from build123d import *

# Parameters (mm, degrees)
SKETCH1_R           = 200
SKETCH1_R_2         = 12.7
BOSS_EXTRUDE1_DEPTH = 30
SKETCH2_R           = 186.107166766
CUT_EXTRUDE3_DEPTH  = 8


with BuildPart() as part:
    # Sketch1 → Boss-Extrude1 (new body)
    with BuildSketch(Plane.XY):
        Circle(SKETCH1_R)
        Circle(SKETCH1_R_2, mode=Mode.SUBTRACT)
        with BuildLine():
            Line((5.373353022, 179.700844592), (5.373353022, 22.746286446))
            ThreePointArc((5.373353022, 22.746286446), (6.167799965, 20.041970731), (8.298682417, 18.197029157))
            ThreePointArc((8.298682417, 18.197029157), (10.179469581, 17.215644021), (11.945725569, 16.040562354))
            Line((11.945725569, 16.040562354), (42.519793553, 175.083108319))
            ThreePointArc((42.519793553, 175.083108319), (41.777732217, 178.788808127), (38.654411976, 180.916656046))
            ThreePointArc((38.654411976, 180.916656046), (24.73012638, 183.339632511), (10.661501717, 184.69253472))
            ThreePointArc((10.661501717, 184.69253472), (6.941206716, 183.336827504), (5.373353022, 179.700844592))
        make_face(mode=Mode.SUBTRACT)
        with BuildLine():
            Line((88.269014329, 156.620073998), (15.3285942, 17.643714734))
            ThreePointArc((15.3285942, 17.643714734), (14.775283856, 14.879964185), (15.804699463, 12.256079099))
            ThreePointArc((15.804699463, 12.256079099), (17.013981377, 10.51306034), (18.031835705, 8.651757112))
            Line((18.031835705, 8.651757112), (119.01458488, 135.268459916))
            ThreePointArc((119.01458488, 135.268459916), (120.079646768, 138.894547239), (118.302944275, 142.23014229))
            ThreePointArc((118.302944275, 142.23014229), (107.099615, 150.846519571), (95.271191525, 158.582470864))
            ThreePointArc((95.271191525, 158.582470864), (91.347005342, 159.110959035), (88.269014329, 156.620073998))
        make_face(mode=Mode.SUBTRACT)
        with BuildLine():
            Line((150.94330821, 97.659531928), (21.772239177, 8.499180607))
            ThreePointArc((21.772239177, 8.499180607), (19.997928277, 6.309137168), (19.690050329, 3.507409022))
            ThreePointArc((19.690050329, 3.507409022), (19.950795079, 1.402061232), (19.987069587, -0.719061419))
            Line((19.987069587, -0.719061419), (168.244569093, 64.465437509))
            ThreePointArc((168.244569093, 64.465437509), (170.872761362, 67.181219439), (170.849697746, 70.960416994))
            ThreePointArc((170.849697746, 70.960416994), (164.933872514, 83.796286896), (158.055399498, 96.14307406))
            ThreePointArc((158.055399498, 96.14307406), (154.826305895, 98.434687345), (150.94330821, 97.659531928))
        make_face(mode=Mode.SUBTRACT)
        with BuildLine():
            Line((179.038309244, 16.326368018), (23.228126543, -2.592413372))
            ThreePointArc((23.228126543, -2.592413372), (20.639288331, -3.707037141), (19.064647955, -6.044766194))
            ThreePointArc((19.064647955, -6.044766194), (18.317122063, -8.030133208), (17.363506697, -9.925151645))
            Line((17.363506697, -9.925151645), (178.931750093, -21.10583974))
            ThreePointArc((178.931750093, -21.10583974), (182.520985567, -19.922516113), (184.256844426, -16.565484669))
            ThreePointArc((184.256844426, -16.565484669), (184.983767504, -2.450665253), (184.631020219, 11.678457638))
            ThreePointArc((184.631020219, 11.678457638), (182.836765627, 15.208215052), (179.038309244, 16.326368018))
        make_face(mode=Mode.SUBTRACT)
        with BuildLine():
            Line((166.117791277, -68.746970051), (19.362730047, -13.090116689))
            ThreePointArc((19.362730047, -13.090116689), (16.552436159, -12.873973916), (14.071764489, -14.212158322))
            ThreePointArc((14.071764489, -14.212158322), (12.487217127, -15.622720904), (10.762173676, -16.85750924))
            Line((10.762173676, -16.85750924), (148.627823508, -101.842023456))
            ThreePointArc((148.627823508, -101.842023456), (152.355851595, -102.462243316), (155.452968583, -100.29643343))
            ThreePointArc((155.452968583, -100.29643343), (162.656110654, -88.136199526), (168.909899254, -75.461552688))
            ThreePointArc((168.909899254, -75.461552688), (168.961525775, -71.502276031), (166.117791277, -68.746970051))
        make_face(mode=Mode.SUBTRACT)
        with BuildLine():
            Line((115.141689264, -138.071205772), (11.061565443, -20.589032025))
            ThreePointArc((11.061565443, -20.589032025), (8.673620341, -19.091638415), (5.855209362, -19.123716253))
            ThreePointArc((5.855209362, -19.123716253), (3.796641234, -19.636331514), (1.695356364, -19.928014623))
            Line((1.695356364, -19.928014623), (84.275053717, -159.247426929))
            ThreePointArc((84.275053717, -159.247426929), (87.28782811, -161.529105379), (91.036691049, -161.050677996))
            ThreePointArc((91.036691049, -161.050677996), (103.065899072, -153.630792644), (114.493555954, -145.314230704))
            ThreePointArc((114.493555954, -145.314230704), (116.379236576, -141.832457371), (115.141689264, -138.071205772))
        make_face(mode=Mode.SUBTRACT)
        with BuildLine():
            Line((37.788013848, -175.764992189), (0.226329502, -23.37124825))
            ThreePointArc((0.226329502, -23.37124825), (-1.192217369, -20.935638632), (-3.702703668, -19.654261257))
            ThreePointArc((-3.702703668, -19.654261257), (-5.76369941, -19.151495219), (-7.75984666, -18.433252014))
            Line((-7.75984666, -18.433252014), (0.615884744, -180.171164031))
            ThreePointArc((0.615884744, -180.171164031), (2.223215138, -183.591596036), (5.765004707, -184.910153103))
            ThreePointArc((5.765004707, -184.910153103), (19.864532092, -183.930422619), (33.848118782, -181.877169691))
            ThreePointArc((33.848118782, -181.877169691), (37.135866798, -179.670531994), (37.788013848, -175.764992189))
        make_face(mode=Mode.SUBTRACT)
        with BuildLine():
            Line((-48.222440145, -173.193137093), (-10.660755799, -20.799393154))
            ThreePointArc((-10.660755799, -20.799393154), (-10.784932447, -17.98353634), (-12.412371909, -15.682251866))
            ThreePointArc((-12.412371909, -15.682251866), (-14.00364598, -14.279282169), (-15.43736233, -12.715653514))
            Line((-15.43736233, -12.715653514), (-83.184376002, -159.819858752))
            ThreePointArc((-83.184376002, -159.819858752), (-83.350709631, -163.59546456), (-80.827374738, -166.408940544))
            ThreePointArc((-80.827374738, -166.408940544), (-67.887559797, -172.093809374), (-54.551514489, -176.77424096))
            ThreePointArc((-54.551514489, -176.77424096), (-50.614882527, -176.348253002), (-48.222440145, -173.193137093))
        make_face(mode=Mode.SUBTRACT)
        with BuildLine():
            Line((-123.185714244, -130.944821493), (-19.105590424, -13.462647747))
            ThreePointArc((-19.105590424, -13.462647747), (-17.906949474, -10.911622598), (-18.278515332, -8.117627564))
            ThreePointArc((-18.278515332, -8.117627564), (-19.035526018, -6.135857658), (-19.578364331, -4.085052034))
            Line((-19.578364331, -4.085052034), (-147.928098686, -102.855749871))
            ThreePointArc((-147.928098686, -102.855749871), (-149.829991307, -106.121583693), (-148.903176705, -109.785445151))
            ThreePointArc((-148.903176705, -109.785445151), (-140.087429871, -120.832578356), (-130.454053207, -131.174463985))
            ThreePointArc((-130.454053207, -131.174463985), (-126.77037224, -132.626714474), (-123.185714244, -130.944821493))
        make_face(mode=Mode.SUBTRACT)
        with BuildLine():
            Line((-169.928625759, -58.698625345), (-23.173564529, -3.041771983))
            ThreePointArc((-23.173564529, -3.041771983), (-20.926700178, -1.339987618), (-19.957271172, 1.306647384))
            ThreePointArc((-19.957271172, 1.306647384), (-19.706596449, 3.413217897), (-19.234199009, 5.481385637))
            Line((-19.234199009, 5.481385637), (-178.783276688, -22.328628241))
            ThreePointArc((-178.783276688, -22.328628241), (-181.985027623, -24.336526905), (-182.867055368, -28.011427332))
            ThreePointArc((-182.867055368, -28.011427332), (-180.194957997, -41.890059828), (-176.471140477, -55.524198135))
            ThreePointArc((-176.471140477, -55.524198135), (-173.884297422, -58.521993984), (-169.928625759, -58.698625345))
        make_face(mode=Mode.SUBTRACT)
        with BuildLine():
            Line((-177.742936974, 26.994718474), (-21.932754273, 8.075937085))
            ThreePointArc((-21.932754273, 8.075937085), (-19.152396066, 8.538622377), (-17.064056697, 10.431585164))
            ThreePointArc((-17.064056697, 10.431585164), (-15.863123123, 12.180366365), (-14.483710491, 13.792103916))
            Line((-14.483710491, 13.792103916), (-168.681360573, 63.313713031))
            ThreePointArc((-168.681360573, 63.313713031), (-172.449487267, 63.02373491), (-174.938295432, 60.179670914))
            ThreePointArc((-174.938295432, 60.179670914), (-179.021992831, 46.648966577), (-182.060816172, 32.845992368))
            ThreePointArc((-182.060816172, 32.845992368), (-181.163425598, 28.98941006), (-177.742936974, 26.994718474))
        make_face(mode=Mode.SUBTRACT)
        with BuildLine():
            Line((-144.838483363, 106.503897613), (-15.667414331, 17.343546292))
            ThreePointArc((-15.667414331, 17.343546292), (-12.990508827, 16.461136886), (-10.261672478, 17.166772497))
            ThreePointArc((-10.261672478, 17.166772497), (-8.385599461, 18.157139689), (-6.415178447, 18.943217401))
            Line((-6.415178447, 18.943217401), (-119.936577581, 134.45164566))
            ThreePointArc((-119.936577581, 134.45164566), (-123.40784762, 135.946018575), (-126.933280248, 134.584331798))
            ThreePointArc((-126.933280248, 134.584331798), (-136.837246557, 124.50127692), (-145.942552953, 113.691561858))
            ThreePointArc((-145.942552953, 113.691561858), (-146.940196225, 109.85968962), (-144.838483363, 106.503897613))
        make_face(mode=Mode.SUBTRACT)
        with BuildLine():
            Line((-78.753278707, 161.61431732), (-5.812858579, 22.637958056))
            ThreePointArc((-5.812858579, 22.637958056), (-3.852652568, 20.612603314), (-1.10846276, 19.969259133))
            ThreePointArc((-1.10846276, 19.969259133), (1.01296398, 19.974331127), (3.122993668, 19.75466807))
            Line((3.122993668, 19.75466807), (-43.715770058, 174.788326586))
            ThreePointArc((-43.715770058, 174.788326586), (-46.094957309, 177.724707712), (-49.849380271, 178.157344184))
            ThreePointArc((-49.849380271, 178.157344184), (-63.304736163, 173.831845124), (-76.39060965, 168.491764657))
            ThreePointArc((-76.39060965, 168.491764657), (-79.054738718, 165.562438241), (-78.753278707, 161.61431732))
        make_face(mode=Mode.SUBTRACT)
    extrude(amount=BOSS_EXTRUDE1_DEPTH)

    # Sketch2 → Cut-Extrude3 (cut)
    with BuildSketch(Plane.XY):
        Circle(SKETCH2_R)
    cut_extrude3 = extrude(amount=CUT_EXTRUDE3_DEPTH, mode=Mode.SUBTRACT)

    # Mirror1: Cut-Extrude3 across plane
    add(cut_extrude3.mirror(Plane.XY.offset(15)), mode=Mode.SUBTRACT)


solid = part.part
Geometry: final body of the model. Coordinates: model frame, mm. A direction names the side the tool comes from. Round coordinates to 2 decimals unless told otherwise and drop trailing zeros. Order: outer loops, then holes, each group sorted by start corner. A loop starts at its lowest first (then second) coordinate and runs counter-clockwise, first axis right, second up. Notation, with made-up numbers: (73.5, -33) -> (104.5, -33) arc R8 ccw to (104.5, -24) -> close; hole circle Ø11 at (-17.75, 8). An arc over 180 degrees is marked (long way). Put each result on its own line as item: value. Start each with the question number.
Q1. Line query: probe 1 along Y at (x, z) = (0, 6.5); probe 2 along Y at (x, z) = (-170, 11); probe 3 along Z at (x, y) = (48.5, 109). Output: solid intervals per line, ascending.
Q2. Pull-direction query (Y, two-part tool) for faces 1 (the cylindrical face through (190.764, 60.075, 14.79)), 2 (the flat face through (-90.503, 38.206, 14.902)), 3 (the flat face through (177, -58, 30)); classes: +Y half, -Y half, draft (parallel to the pull), parting line (faces both ways), or undercut.
Q3. First-contact query: pin 1 (3 mm diameter, centred on y = 45.5, z = 11, fed in from +X); pin 2 (5 mm diameter, centred on x = 59.5, z = 5.5, fed in from +Y); pin 3 (15.5 mm diameter, centred on y = 108, z = 13.5, fed in from +X). Flat tips, straight axial feed; report the tip coordinate or a pass-through.
Q4. Section A-A on y = -80.5. Give the number of separate pieces and of enclosed holes in the cut face, and give its area (3 significant figures).
Q5. Reachability of faces 4 (the flat face through (-48.837, -85.238, 14.902)), 5 (the cylindrical face through (177.513, 55.902, 3.944)), 6 (the flat face through (177, -58, 0)), 7 (the flat face through (39, 3, 22)) from +Z, -Z, +X, -X, +Y, -Y: full face, straight path, thin tool, end or side. Return the list, or none.
Q6. Section B-B on x = -104.5. Return the cut outline in (y, z).
Ans:
1. probe 1: y = -200 to -186.11, 186.11 to 200
1. probe 2: y = -105.36 to -58.73, -20.8 to 26.05, 63.55 to 105.36
1. probe 3: z = 8 to 22
2. face 1: parting line
2. face 2: undercut
2. face 3: draft
3. pin 1: stops at x = 195.1
3. pin 2: stops at y = 191.71
3. pin 3: stops at x = 173.06
4. separate pieces: 6
4. enclosed holes: 0
4. area: 3,380 mm2
5. face 4: +Z, -Z
5. face 5: -Z
5. face 6: -Z, +X, -X, +Y, -Y
5. face 7: +Z
6. outline: (-170.53, 0) -> (-154, 0) -> (-154, 8) -> (-109.85, 8) -> (-109.85, 22) -> (-154, 22) -> (-154, 30) -> (-170.53, 30) -> close; (-69.44, 8) -> (-33.88, 8) -> (-33.88, 22) -> (-69.44, 22) -> close; (-9.38, 8) -> (18.1, 8) -> (18.1, 22) -> (-9.38, 22) -> close; (42.7, 8) -> (78.66, 8) -> (78.66, 22) -> (42.7, 22) -> close; (118.74, 8) -> (154, 8) -> (154, 0) -> (170.53, 0) -> (170.53, 30) -> (154, 30) -> (154, 22) -> (118.74, 22) -> close
